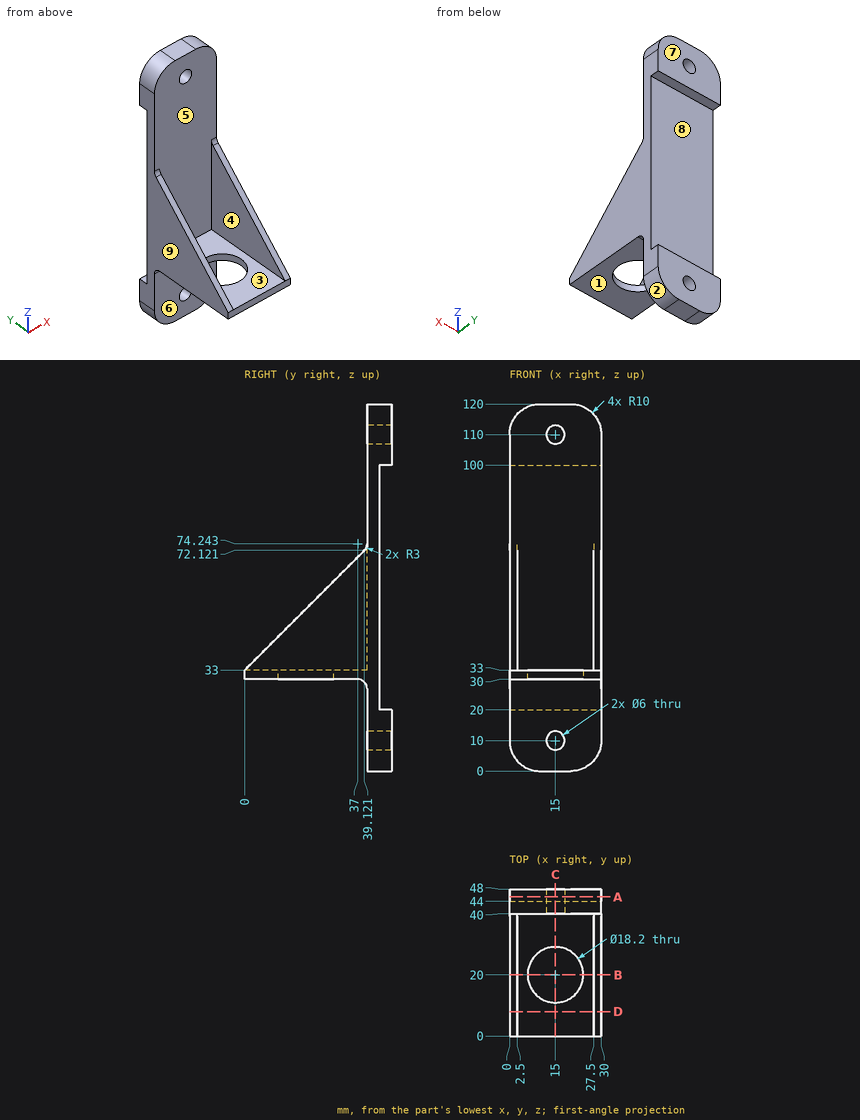
Study the drawing (mm; zero at the part's minimum x, y, z) and answer. A direction names the side the tool comes from. Give positions to 0.01 mm unless a question says otherwise; leave off trailing zeros. Order: outer loops, then holes, each group sorted by start corner. A loop starts at its lowest first (then second) coordinate and runs counter-clockwise, first axis right, second up. Notation, with made-up numbers: (-7, 0.5) - (5, 0.5) arc R14 cw to (5, 4.5) - close; hole circle Ø11 at (23.5, -28). An arc over 180 degrees is marked (long way). Answer in a Markdown table with one row per item. Add a question column.
Q1. Given P1, Ø12.5, axis at x = 9.5, y = 18, coming from the +Z side; P2, Ø8, axis at x = 11.5, z = 9, coming from the -Y side; P3, Ø2, axis at x = 27, y = 16.5, coming from the +Z side (1 decimal), each flat-ended and moving along its own axis, determine where each tip first touches the part or whether it passes through.
Q2. The part is cut by section D-D (y = 8). Determine the outline of the cut face in (x, z), then the cut area to 3 significant figures.
Q3. Which of the six approach directions +Z, -Z, +X, -X, +Y, -Y give full straight-line access (tool end or side, diameter ignored) to the marked faces 5, 6, 7, 8 and 9?
Q4. The part is cut by section C-C (x = 15). Determine the outline of the cut face in (y, z).
Q5. The part is cut by section B-B (y = 20). Determine the outline of the cut face in (x, z), then the cut area to 3 significant figures.
Q6. The part is cut by section A-A (y = 45.5). Determine the outline of the cut face in (x, z), then the cut area to 3 significant figures.
Q7. Find the intervals of material crossed by line 1 along X through (y, z) = (37, 54); line 2 along X through (y, z) = (44, 10); line 3 along Y through (x, z) = (25.75, 111), in increasing order. Write a range as [from, to].
Q8. For a pull along X with two mould halves and no side action, classify the marked faces 1, 2, 3 and 4 as released by +X, released by -X, zero draft, split by the parting line, or undercut.
Determined:
| question | item | result |
|---|---|---|
| 1 | P1 | stops at z = 33 |
| 1 | P2 | stops at y = 40 |
| 1 | P3 | stops at z = 50.4 |
| 2 | outline | (0, 30) - (30, 30) - (30, 41) - (27.5, 41) - (27.5, 33) - (2.5, 33) - (2.5, 41) - (0, 41) - close |
| 2 | area | 130 mm² |
| 3 | face 5 | +Z, -Y |
| 3 | face 6 | -Z, +X, -X, -Y |
| 3 | face 7 | +Z, -Z, +X, -X, +Y |
| 3 | face 8 | +X, -X, +Y |
| 3 | face 9 | +Z, -Z, -X, +Y, -Y |
| 4 | outline | (0, 30) - (10.9, 30) - (10.9, 33) - (0, 33) - close; (29.1, 30) - (37, 30) arc R3 cw to (40, 27) - (40, 13) - (48, 13) - (48, 20) - (44, 20) - (44, 100) - (48, 100) - (48, 107) - (40, 107) - (40, 33) - (29.1, 33) - close; (40, 0) - (48, 0) - (48, 7) - (40, 7) - close; (40, 113) - (48, 113) - (48, 120) - (40, 120) - close |
| 5 | outline | (0, 30) - (5.9, 30) - (5.9, 33) - (2.5, 33) - (2.5, 53) - (0, 53) - close; (24.1, 30) - (30, 30) - (30, 53) - (27.5, 53) - (27.5, 33) - (24.1, 33) - close |
| 5 | area | 135 mm² |
| 6 | outline | (0, 10) arc R10 ccw to (10, 0) - (20, 0) arc R10 ccw to (30, 10) - (30, 20) - (0, 20) - close; (0, 100) - (30, 100) - (30, 110) arc R10 ccw to (20, 120) - (10, 120) arc R10 ccw to (0, 110) - close; hole circle Ø6 at (15, 10); hole circle Ø6 at (15, 110) |
| 6 | area | 1,060 mm² |
| 7 | line 1 | x = [0, 2.5], [27.5, 30] |
| 7 | line 2 | x = [0, 12], [18, 30] |
| 7 | line 3 | y = [40, 48] |
| 8 | face 1 | zero draft |
| 8 | face 2 | released by +X |
| 8 | face 3 | undercut |
| 8 | face 4 | undercut |
